from build123d import *

# Parameters (mm, degrees)
F0_W     = 150
F0_H     = 150
F0_W_2   = 140
F0_H_2   = 140
F1_DEPTH = 25
F2_DEPTH = 5
F3_R     = 2.5
F4_DEPTH = 6
F5_W     = 5
F5_H     = 5
F6_DEPTH = 12.85037


with BuildPart() as f1:
    # F0 (on Top) → F1 (new body)
    with BuildSketch(Plane.XY):
        with Locations((9.114077, -2.272729)):
            Rectangle(F0_W, F0_H)
        with Locations((9.114077, -2.272729)):
            Rectangle(F0_W_2, F0_H_2, mode=Mode.SUBTRACT)
    extrude(amount=F1_DEPTH)

    # F0 (on Top) → F2 (join)
    with BuildSketch(Plane.XY):
        with Locations((9.114077, -2.272729)):
            Rectangle(F0_W_2, F0_H_2)
    extrude(amount=F2_DEPTH)

    # F3 (on face) → F4 (cut)
    with BuildSketch(Plane(origin=(0, 72.727271, 0), x_dir=(-1, 0, 0), z_dir=(0, 1, 0))):
        with Locations((56.684904, 12.5)):
            Circle(F3_R)
    extrude(amount=-F4_DEPTH, mode=Mode.SUBTRACT)

    # F5 (on face) → F6 (cut)
    with BuildSketch(Plane.XY.offset(25)):
        with Locations((-56.685923, 70.227271)):
            Rectangle(F5_W, F5_H)
    extrude(amount=-F6_DEPTH, mode=Mode.SUBTRACT)


solid = f1.part
The listing builds one solid part. Answer for the finished solid, in the listing's coordinates (mm). A direction names the side the tool comes from. Coordinates: 2 decimals unless noted, no trailing zeros. Write each loop counter-clockwise with the first axis right and the second up, starting at its lowest first coordinate (ties: lowest second). Pieces come first, ordered by that corner, then holes. Notation, with made-up numbers: M -18,-39.75 L 9,-39.75 A23 cw 9,-5.75 Z; hole C 85.5,-4.75 d1. An arc over 180 degrees is marked long. Put each result on its own line as item: value. Start each with the question number.
1. A cutting plane is placed at B-B on y = 8. Write down the section's boundary in (x, z), then the cut area to 3 significant figures.
2. A cutting plane is placed at C-C on x = -48. Write down the section's boundary in (y, z), then the cut area to 3 significant figures.
3. A cutting plane is placed at A-A on z = 8.25. Write down the section's boundary in (x, y), then the cut area to 3 significant figures.
4. Which of the six approach directions +Z, -Z, +X, -X, +Y, -Y give full straight-line access (tool end or side, diameter ignored) to faces 1 (the cylindrical face through (-56.6, 70.3, 10)), 2 (the flat face through (-60.886, -3, 15)), 3 (the flat face through (84.114, -3, 12))?
5. Consider line 1 (Y direction, x = 16, z = 22); line 2 (X direction, y = -19, z = 13); line 3 (Z direction, x = 57.5, y = -6.5). Determine where each line is inside the solid, lowest interval first. Write a range as from..to.
6. For a pull along Y with two mould halves and no side action, classify faces 4 (the flat face through (-59.186, 70, 19)), 5 (the flat face through (8, 72.727, 12)), 6 (the flat face through (8, 67.727, 15)) as pulls with the +Y half, pulls with the -Y half, needs draft (parallel to the pull), parting line crosses it, or undercut.
Resolved:
1. outline: M -65.89,0 L 84.11,0 L 84.11,25 L 79.11,25 L 79.11,5 L -60.89,5 L -60.89,25 L -65.89,25 Z
1. area: 950 mm2
2. outline: M -77.27,0 L 72.73,0 L 72.73,25 L 67.73,25 L 67.73,5 L -72.27,5 L -72.27,25 L -77.27,25 Z
2. area: 950 mm2
3. outline: M -65.89,-77.27 L 84.11,-77.27 L 84.11,72.73 L -65.89,72.73 Z; hole M -60.89,-72.27 L 79.11,-72.27 L 79.11,67.73 L -60.89,67.73 Z
3. area: 2,900 mm2
4. face 1: +Z, +Y
4. face 2: +Z
4. face 3: +Z, -Z, +X, +Y, -Y
5. line 1: y = -77.27..-72.27, 67.73..72.73
5. line 2: x = -65.89..-60.89, 79.11..84.11
5. line 3: z = 0..5
6. face 4: needs draft
6. face 5: pulls with the +Y half
6. face 6: undercut
